```python
from build123d import *

# Parameters (mm, degrees)
SKETCH1_W           = 8.5
SKETCH1_H           = 3.9
BOSS_EXTRUDE1_DEPTH = 4
SKETCH2_W           = 1.5
SKETCH2_H           = 1.5
BOSS_EXTRUDE2_DEPTH = 4
CHAMFER1_SIZE       = 0.2
SKETCH3_W           = 2.1
SKETCH3_H           = 1.5
CUT_EXTRUDE1_DEPTH  = 0.2
SKETCH4_W           = 0.5
SKETCH4_H           = 0.3
BOSS_EXTRUDE3_DEPTH = 2


with BuildPart() as part:
    # Sketch1 → Boss-Extrude1 (new body)
    with BuildSketch(Plane.XY):
        Rectangle(SKETCH1_W, SKETCH1_H)
    extrude(amount=BOSS_EXTRUDE1_DEPTH)

    # Sketch2 → Boss-Extrude2 (add)
    with BuildSketch(Plane.XY.offset(4)):
        with Locations((-1.15, 0)):
            Rectangle(SKETCH2_W, SKETCH2_H)
    extrude(amount=BOSS_EXTRUDE2_DEPTH)

    # Chamfer1
    chamfer1_edges = [part.edges().sort_by_distance(p)[0] for p in [
        (-0.4, 0, 8),
        (-1.15, 0.75, 8),
        (-1.9, 0, 8),
        (-1.15, -0.75, 8),
    ]]
    chamfer(chamfer1_edges, length=CHAMFER1_SIZE)

    # Sketch3 → Cut-Extrude1 (cut)
    with BuildSketch(Plane.XY.offset(4)):
        with Locations((0.65, 0)):
            Rectangle(SKETCH3_W, SKETCH3_H)
    extrude(amount=-CUT_EXTRUDE1_DEPTH, mode=Mode.SUBTRACT)

    # Sketch4 → Boss-Extrude3 (add)
    with BuildSketch(Plane(origin=(0, 0, 0), x_dir=(-1, 0, 0), z_dir=(0, 0, -1))):
        Rectangle(SKETCH4_W, SKETCH4_H)
        with Locations((2.5, 0)):
            Rectangle(SKETCH4_W, SKETCH4_H)
        with Locations((-2.5, 0)):
            Rectangle(SKETCH4_W, SKETCH4_H)
    extrude(amount=BOSS_EXTRUDE3_DEPTH)


solid = part.part
```
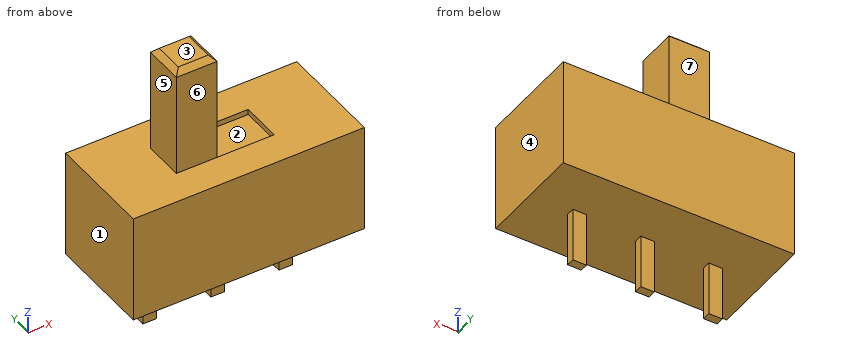
The listing builds one solid part. Answer for the finished solid, in the listing's coordinates (mm). Face numbers are marked on the shaded views. A direction names the side the tool comes from. Round coordinates to 2 decimals unless told otherwise and drop trailing zeros. Loops run counter-clockwise (first coordinate to the right, second up) from the corner with the lowest first, then second, coordinate; pieces in that order, holes last.
1) Consider line 1 (Z direction, x = -0.25, y = 0.55); line 2 (Z direction, x = -2, y = -1.65); line 3 (X direction, y = 0, z = 7.75). Determine where each line is inside the solid, lowest interval first.
Outcome:
line 1: z = 0 to 3.8
line 2: z = 0 to 4
line 3: x = -1.9 to -0.4
2) For the marked faces 4, 5, 6 and 7, determine the directions among +Z, -Z, +X, -X, +Y, -Y from which every point of the face is accessible in a straight line to the end or side of a thin tool.
Outcome:
face 4: +Z, -Z, +X, +Y, -Y
face 5: +Z, -X, +Y, -Y
face 6: +Z, +X, -X, -Y
face 7: +Z, +X, -X, +Y
3) For a pull along X with two mould halves and no side action, classify the marked faces 1, 2 and 3 as released by +X, released by -X, zero draft, split by the parting line, or undercut.
Outcome:
face 1: released by -X
face 2: undercut
face 3: zero draft
4) A cutting plane is placed at A-A on z = -1. Determine the outline of the cut face in (x, y), plus the area to 3 significant figures.
Outcome:
outline: (-2.75, -0.15) - (-2.25, -0.15) - (-2.25, 0.15) - (-2.75, 0.15) - close; (-0.25, -0.15) - (0.25, -0.15) - (0.25, 0.15) - (-0.25, 0.15) - close; (2.25, -0.15) - (2.75, -0.15) - (2.75, 0.15) - (2.25, 0.15) - close
area: 0.450 mm2
5) A cutting plane is placed at C-C on y = 0.35. Determine the outline of the cut face in (x, z).
Outcome:
outline: (-4.25, 0) - (4.25, 0) - (4.25, 4) - (1.7, 4) - (1.7, 3.8) - (-0.4, 3.8) - (-0.4, 7.8) - (-0.6, 8) - (-1.7, 8) - (-1.9, 7.8) - (-1.9, 4) - (-4.25, 4) - close
6) Given P1, Ø1.2, axis at x = 2, y = -0.5, coming from the +Z side; P2, Ø1.5, axis at x = -2.5, y = -0.5, coming from the +Z side; P3, Ø0.6, axis at x = 0, z = -1.5, coming from the -Y side, each flat-ended and moving along its own axis, determine where each tip first touches the part or whether it passes through.
Outcome:
P1: stops at z = 4
P2: stops at z = 7.95
P3: stops at y = -0.15
7) A cutting plane is placed at B-B on x = 2.5. Determine the outline of the cut face in (y, z).
Outcome:
outline: (-1.95, 0) - (-0.15, 0) - (-0.15, -2) - (0.15, -2) - (0.15, 0) - (1.95, 0) - (1.95, 4) - (-1.95, 4) - close
8) A cutting plane is placed at D-D on z = 6. Determine the outline of the cut face in (x, y).
Outcome:
outline: (-1.9, -0.75) - (-0.4, -0.75) - (-0.4, 0.75) - (-1.9, 0.75) - close
